from build123d import *

# Parameters (mm, degrees)
ESQUISSE1_R             = 16.1
BOSS_EXTRU_1_DEPTH      = 8
ESQUISSE2_R             = 1.25
ENL_V_MAT_EXTRU_1_DEPTH = 15


with BuildPart() as part:
    # Esquisse1 → Boss.-Extru.1 (new body)
    with BuildSketch(Plane.XY):
        with BuildLine():
            Line((-20, 0), (-20, -26))
            Line((-20, -26), (20, -26))
            Line((20, -26), (20, 0))
            ThreePointArc((20, 0), (0, 20), (-20, 0))
        make_face()
        Circle(ESQUISSE1_R, mode=Mode.SUBTRACT)
    extrude(amount=BOSS_EXTRU_1_DEPTH)

    # Esquisse2 → Enlèv. mat.-Extru.1 (cut)
    with BuildSketch(Plane.XZ.offset(26)):
        with Locations((-16, 4)):
            Circle(ESQUISSE2_R)
        with Locations((16, 4)):
            Circle(ESQUISSE2_R)
    extrude(amount=-ENL_V_MAT_EXTRU_1_DEPTH, mode=Mode.SUBTRACT)


solid = part.part
Can you work these out from the model? Positions are in its coordinate system, mm. A direction names the side the tool comes from. Round coordinates to 2 decimals unless told otherwise and drop trailing zeros. Order: outer loops, then holes, each group sorted by start corner. A loop starts at its lowest first (then second) coordinate and runs counter-clockwise, first axis right, second up. Notation, with made-up numbers: (15, 66.25) -> (27, 66.25) arc R11 cw to (27, 75.25) -> close; hole circle Ø8 at (39, -12). An arc over 180 degrees is marked (long way). Write each question's results on one line, items separated by ' | '. Start each with the question number.
Item 1: Thinking about a two-plate mould opening in X: for faces 3 (the cylindrical face through (15.73, -18.6, 2.78)), 4 (the flat face through (20, -13, 4)), 5 (the flat face through (0, -18, 8)), which applies, +X half, -X half, draft (parallel to the pull), parting line (faces both ways), or undercut?
Item 2: Will these pins go through, and if not, where does the flat tip stop? pin 1 (8 mm diameter, centred on x = 8.5, y = -17, fed in from -Z); pin 2 (19.5 mm diameter, centred on x = 0, y = 0, fed in from +Z); pin 3 (1.5 mm diameter, centred on y = 3.5, z = 2.5, fed in from -X); pin 4 (2 mm diameter, centred on x = 16, z = 4, fed in from -Y).
Item 3: If we section it at A-A, the plane x = 0: Write out the boundary of the cut face in (y, z).
Item 4: Please list where these lines run through material, in increasing order: L1, parallel to Z at x = 16, y = -15; L2, parallel to Y at x = 0, z = 4; L3, parallel to Y at x = -9, z = 5.75.
Item 5: Which directions (+Z, -Z, +X, -X, +Y, -Y) give clear straight access to the entire face, cutting with the end or side of a thin tool? Please do faces 1 (the flat face through (-20, -13, 4)), 2 (the flat face through (16, -11, 4)).
Item 6: If we section it at C-C, the plane z = 4: Write out the boundary of the cut face in (x, y).
Item 7: If we section it at B-B, the plane y = -10.5: Write out the boundary of the cut face in (x, z), then the cut area to 3 significant figures.
Item 8: If we section it at D-D, the plane z = 0.5: Write out the boundary of the cut face in (x, y), then the cut area to 3 significant figures.
Results:
1) face 3: undercut | face 4: +X half | face 5: draft
2) pin 1: stops at z = 0 | pin 2: passes through | pin 3: stops at x = -19.81 | pin 4: stops at y = -11
3) outline: (-26, 0) -> (-16.1, 0) -> (-16.1, 8) -> (-26, 8) -> close; (16.1, 0) -> (20, 0) -> (20, 8) -> (16.1, 8) -> close
4) L1: z = 0 to 2.75, 5.25 to 8 | L2: y = -26 to -16.1, 16.1 to 20 | L3: y = -26 to -13.35, 13.35 to 17.86
5) face 1: +Z, -Z, -X, +Y, -Y | face 2: -Y
6) outline: (-20, -26) -> (-17.25, -26) -> (-17.25, -11) -> (-14.75, -11) -> (-14.75, -26) -> (14.75, -26) -> (14.75, -11) -> (17.25, -11) -> (17.25, -26) -> (20, -26) -> (20, 0) arc R20 ccw to (-20, 0) -> close; hole circle Ø32.2 at (0, 0)
7) outline: (-20, 0) -> (-12.2, 0) -> (-12.2, 8) -> (-20, 8) -> close; (12.2, 0) -> (20, 0) -> (20, 8) -> (12.2, 8) -> close | area: 125 mm2
8) outline: (-20, -26) -> (20, -26) -> (20, 0) arc R20 ccw to (-20, 0) -> close; hole circle Ø32.2 at (0, 0) | area: 854 mm2
